Geometry: see drawing. Coordinates: mm, zero at the bounding-box minimum. Coordinates: 2 decimals unless noted, no trailing zeros. Write each loop counter-clockwise with the first axis right and the second up, starting at its lowest first coordinate (ties: lowest second). Pieces come first, ordered by that corner, then holes.
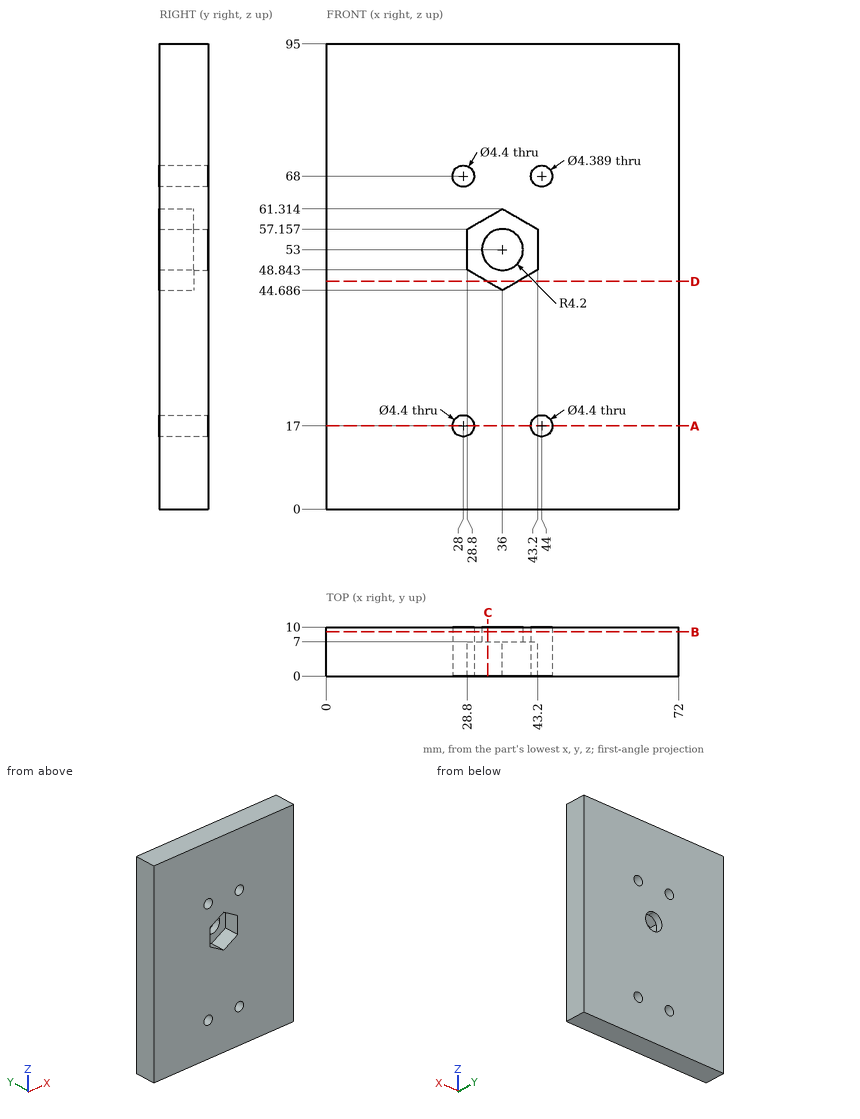
Item 1: Material intervals for probe 1 along X at (y, z) = (7.75, 68) (1 decimal); probe 2 along X at (y, z) = (8.5, 69); probe 3 along X at (y, z) = (3.75, 53), sorted ascending.
Derived:
probe 1: x = 0 to 25.8, 30.2 to 41.8, 46.2 to 72
probe 2: x = 0 to 26.04, 29.96 to 42.05, 45.95 to 72
probe 3: x = 0 to 28.8, 43.2 to 72
Item 2: Pin query (flat end, axial travel): pin 1 (3.5 mm diameter, centred on x = 28, z = 68, fed in from +Y); pin 2 (7 mm diameter, centred on x = 34, z = 52, fed in from -Y). Return the tip coordinate at first contact, or that it passes through.
Derived:
pin 1: passes through
pin 2: stops at y = 7
Item 3: Section C-C, the plane x = 33. Output: boundary loops of the cut face in (y, z), plus the area to 3 significant figures.
Derived:
outline: (0, 0) - (10, 0) - (10, 50.06) - (7, 50.06) - (7, 46.42) - (0, 46.42) - close; (0, 59.58) - (7, 59.58) - (7, 55.94) - (10, 55.94) - (10, 95) - (0, 95) - close
area: 840 mm2
Item 4: Section B-B, the plane y = 9. Output: boundary loops of the cut face in (x, z) (1 decimal).
Derived:
outline: (0, 0) - (72, 0) - (72, 95) - (0, 95) - close; hole circle Ø4.4 at (28, 17); hole circle Ø4.4 at (28, 68); hole circle Ø8.4 at (36, 53); hole circle Ø4.4 at (44, 17); hole circle Ø4.4 at (44, 68)
Item 5: Section A-A, the plane z = 17. Output: boundary loops of the cut face in (x, y), plus the area to 3 significant figures.
Derived:
outline: (0, 0) - (25.8, 0) - (25.8, 10) - (0, 10) - close; (30.2, 0) - (41.8, 0) - (41.8, 10) - (30.2, 10) - close; (46.2, 0) - (72, 0) - (72, 10) - (46.2, 10) - close
area: 632 mm2
Item 6: Section D-D, the plane z = 46.5. Output: boundary loops of the cut face in (x, y).
Derived:
outline: (0, 0) - (32.86, 0) - (32.86, 7) - (39.14, 7) - (39.14, 0) - (72, 0) - (72, 10) - (0, 10) - close
